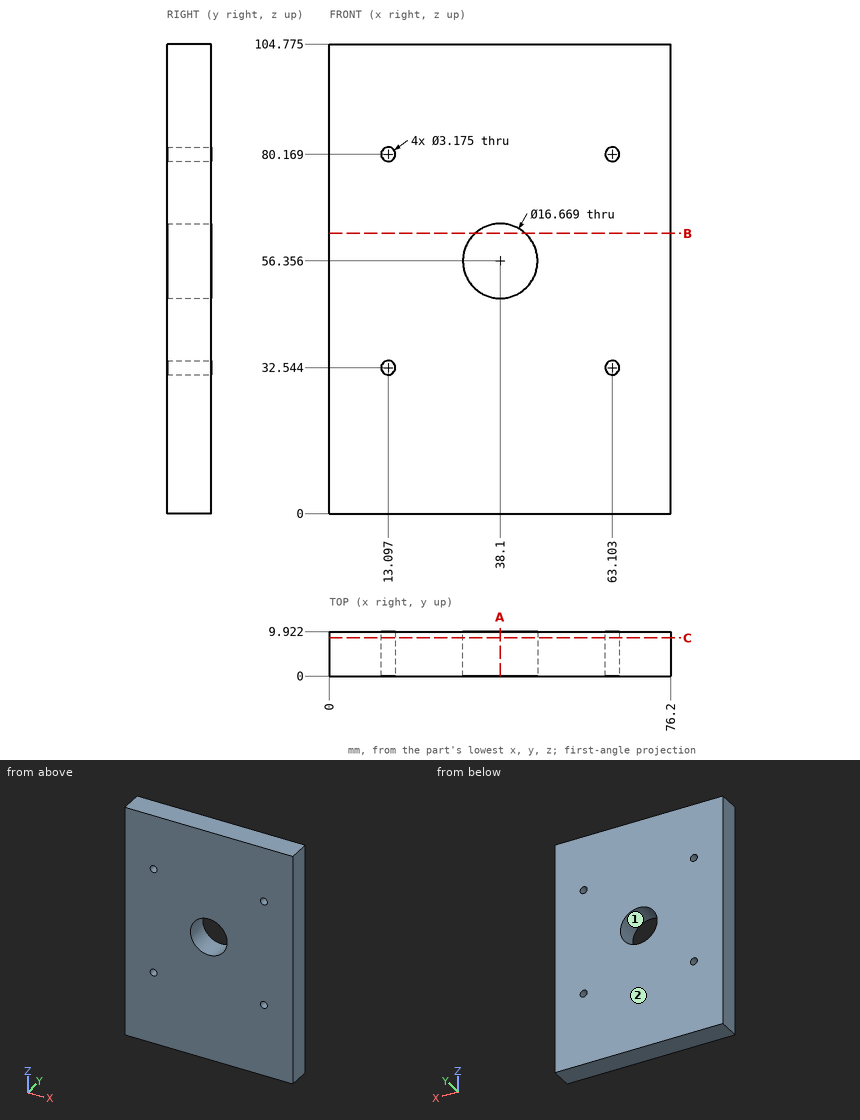
Could you check a few things on this drawing? It's one solid part, dimensions in mm from its lowest x, y, z. Give positions to 0.01 mm unless a question says otherwise; leave off trailing zeros. Loops run counter-clockwise (first coordinate to the right, second up) from the corner with the lowest first, then second, coordinate; pieces in that order, holes last. Notation, with made-up numbers: (-27.5, 7.25) -> (-18.5, 7.25) arc R22 ccw to (-18.5, 32.25) -> close; hole circle Ø6 at (38, -26). An arc over 180 degrees is marked (long way). Use one line per item in the form item = value. Start each with the question number.
1) Please list where these lines run through material, in increasing order: line 1 along Z through (x, y) = (38.1, 6) (1 decimal); line 2 along X through (y, z) = (7.25, 51.5); line 3 along X through (y, z) = (3.75, 51) (1 decimal).
2) Imagine slicing it at B-B (z = 62.5). Please give me the cut outline in (x, y), then the cut area to 3 significant figures.
3) Imagine slicing it at C-C (y = 8.5). Please give me the cut outline in (x, z) (1 decimal), then the cut area to 3 significant figures.
4) Thinking about a two-plate mould opening in X: for the marked faces 1 and 2, which applies, +X half, -X half, draft (parallel to the pull), parting line (faces both ways), or undercut?
5) Imagine slicing it at A-A (x = 38.1). Please give me the cut outline in (y, z) (1 decimal).
Check values:
q1.line_1 = 0 to 48, 64.7 to 104.8
q1.line_2 = 0 to 31.33, 44.87 to 76.2
q1.line_3 = 0 to 31.7, 44.5 to 76.2
q2.outline = (0, 0) -> (32.47, 0) -> (32.47, 9.92) -> (0, 9.92) -> close; (43.73, 0) -> (76.2, 0) -> (76.2, 9.92) -> (43.73, 9.92) -> close
q2.area = 644 mm^2
q3.outline = (0, 0) -> (76.2, 0) -> (76.2, 104.8) -> (0, 104.8) -> close; hole circle Ø3.2 at (13.1, 32.5); hole circle Ø3.2 at (13.1, 80.2); hole circle Ø16.7 at (38.1, 56.4); hole circle Ø3.2 at (63.1, 32.5); hole circle Ø3.2 at (63.1, 80.2)
q3.area = 7,730 mm^2
q4.face_1 = undercut
q4.face_2 = draft
q5.outline = (0, 0) -> (9.9, 0) -> (9.9, 48) -> (0, 48) -> close; (0, 64.7) -> (9.9, 64.7) -> (9.9, 104.8) -> (0, 104.8) -> close
